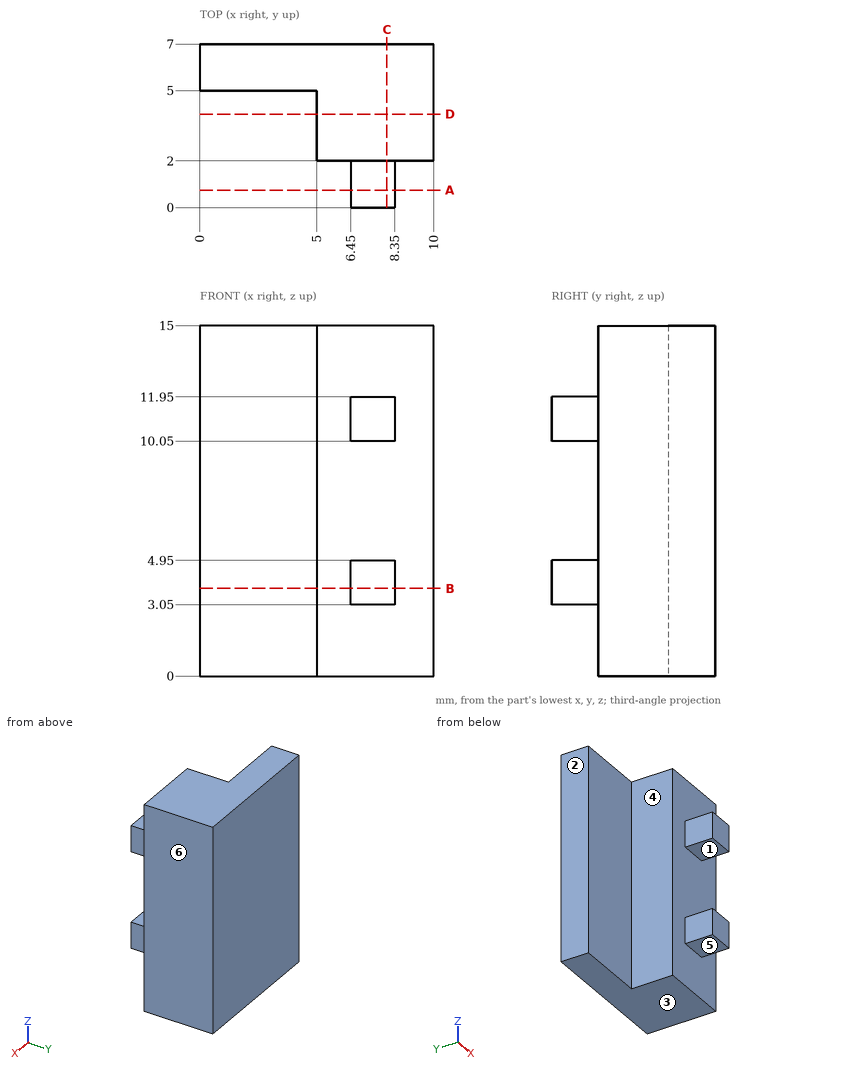
Study the drawing (mm; zero at the part's minimum x, y, z) and answer. A direction names the side the tool comes from. Give positions to 0.01 mm unless a question says otherwise; leave off trailing zeros. Loops run counter-clockwise (first coordinate to the right, second up) from the corner with the lowest first, then second, coordinate; pieces in that order, holes last. Notation, with made-up numbers: (18, -10) -> (34, -10) arc R22 cw to (34, -3) -> close; hole circle Ø11 at (57.25, -14.75). An arc over 180 degrees is marked (long way). Use a Markdown table: item, result. Add a question column.
1) The part is cut by section D-D, the plane y = 4. Determine the outline of the cut face in (x, z).
2) For a pull along Z with two mould halves and no side action, classify the marked faces 1, 2 and 3 as +Z half, -Z half, draft (parallel to the pull), parting line (faces both ways), or undercut.
3) The part is cut by section A-A, the plane y = 0.75. Determine the outline of the cut face in (x, z).
4) Which of the six approach directions +Z, -Z, +X, -X, +Y, -Y give full straight-line access (tool end or side, diameter ignored) to the marked faces 4, 5 and 6?
5) Each of these flat-tipped pins is pushed along its axis until it touches: P1, Ø2, axis at x = 7.5, y = 0.5, coming from the +Z side; P2, Ø0.6, axis at x = 7.5, y = 1, coming from the -Z side; P3, Ø1, axis at y = 1, z = 4, coming from the -X side. Where does it stop, or does it pass through?
6) The part is cut by section C-C, the plane x = 8. Determine the outline of the cut face in (y, z), plus the area to 3 significant figures.
7) The part is cut by section B-B, the plane z = 3.75. Determine the outline of the cut face in (x, y).
8) Consider line 1 along Y through (x, z) = (1.25, 9.5); line 2 along Y through (x, z) = (6.25, 4); line 3 along X through (y, z) = (2.5, 5.5). Determine where each line is inside the solid, lowest interval first.
Reported:
| question | item | result |
|---|---|---|
| 1 | outline | (5, 0) -> (10, 0) -> (10, 15) -> (5, 15) -> close |
| 2 | face 1 | undercut |
| 2 | face 2 | draft |
| 2 | face 3 | -Z half |
| 3 | outline | (6.45, 3.05) -> (8.35, 3.05) -> (8.35, 4.95) -> (6.45, 4.95) -> close; (6.45, 10.05) -> (8.35, 10.05) -> (8.35, 11.95) -> (6.45, 11.95) -> close |
| 4 | face 4 | +Z, -Z, -X, -Y |
| 4 | face 5 | -Z, +X, -X, -Y |
| 4 | face 6 | +Z, -Z, +X, +Y, -Y |
| 5 | P1 | stops at z = 11.95 |
| 5 | P2 | stops at z = 3.05 |
| 5 | P3 | stops at x = 6.45 |
| 6 | outline | (0, 3.05) -> (2, 3.05) -> (2, 0) -> (7, 0) -> (7, 15) -> (2, 15) -> (2, 11.95) -> (0, 11.95) -> (0, 10.05) -> (2, 10.05) -> (2, 4.95) -> (0, 4.95) -> close |
| 6 | area | 82.6 mm^2 |
| 7 | outline | (0, 5) -> (5, 5) -> (5, 2) -> (6.45, 2) -> (6.45, 0) -> (8.35, 0) -> (8.35, 2) -> (10, 2) -> (10, 7) -> (0, 7) -> close |
| 8 | line 1 | y = 5 to 7 |
| 8 | line 2 | y = 2 to 7 |
| 8 | line 3 | x = 5 to 10 |
